```python
from build123d import *

# Parameters (mm, degrees)
SKETCH_1_R      = 2.15
EXTRUDE_1_DEPTH = 6


with BuildPart() as part:
    # 草图1 → 凸台-拉伸1 (new body)
    with BuildSketch(Plane.XY):
        with BuildLine():
            ThreePointArc((-43.896896246, -8.75), (-40.93656063, -9.720556733), (-39.12549448, -12.255434783))
            ThreePointArc((-39.12549448, -12.255434783), (41, 0), (-39.12549448, 12.255434783))
            ThreePointArc((-39.12549448, 12.255434783), (-40.93656063, 9.720556733), (-43.896896246, 8.75))
            Line((-43.896896246, 8.75), (-52, 8.75))
            Line((-52, 8.75), (-52, 30))
            Line((-52, 30), (-47.54, 30))
            ThreePointArc((-47.54, 30), (-44.004466094, 31.464466094), (-42.54, 35))
            Line((-42.54, 35), (-42.54, 37.5))
            ThreePointArc((-42.54, 37.5), (-38.982425028, 42.287422066), (-33.372235985, 40.262198963))
            ThreePointArc((-33.372235985, 40.262198963), (-30.171244586, 38.118753147), (-26.396349665, 38.887436588))
            ThreePointArc((-26.396349665, 38.887436588), (0, 47), (26.396349665, 38.887436588))
            ThreePointArc((26.396349665, 38.887436588), (30.171244586, 38.118753147), (33.372235985, 40.262198963))
            ThreePointArc((33.372235985, 40.262198963), (38.674773042, 42.369526686), (42.499484755, 38.135225128))
            Line((42.499484755, 38.135225128), (46.619156699, 5.971116201))
            ThreePointArc((46.619156699, 5.971116201), (47, 0), (46.619156699, -5.971116201))
            Line((46.619156699, -5.971116201), (42.499484755, -38.135225128))
            ThreePointArc((42.499484755, -38.135225128), (38.674773042, -42.369526686), (33.372235985, -40.262198963))
            ThreePointArc((33.372235985, -40.262198963), (30.171244586, -38.118753147), (26.396349665, -38.887436588))
            ThreePointArc((26.396349665, -38.887436588), (0, -47), (-26.396349665, -38.887436588))
            ThreePointArc((-26.396349665, -38.887436588), (-30.171244586, -38.118753147), (-33.372235985, -40.262198963))
            ThreePointArc((-33.372235985, -40.262198963), (-38.982425028, -42.287422066), (-42.54, -37.5))
            Line((-42.54, -37.5), (-42.54, -35))
            ThreePointArc((-42.54, -35), (-44.004466094, -31.464466094), (-47.54, -30))
            Line((-47.54, -30), (-52, -30))
            Line((-52, -30), (-52, -8.75))
            Line((-52, -8.75), (-43.896896246, -8.75))
        make_face()
        with Locations((37.54, -37.5)):
            Circle(SKETCH_1_R, mode=Mode.SUBTRACT)
        with Locations((-37.54, -37.5)):
            Circle(SKETCH_1_R, mode=Mode.SUBTRACT)
        with Locations((-37.54, 37.5)):
            Circle(SKETCH_1_R, mode=Mode.SUBTRACT)
        with Locations((37.54, 37.5)):
            Circle(SKETCH_1_R, mode=Mode.SUBTRACT)
    extrude(amount=EXTRUDE_1_DEPTH)


solid = part.part
```
The model under review builds one solid part; all positions refer to its coordinate system, in mm. A direction names the side the tool comes from. Give positions to 0.01 mm unless a question says otherwise; leave off trailing zeros. Write each loop counter-clockwise with the first axis right and the second up, starting at its lowest first coordinate (ties: lowest second). Pieces come first, ordered by that corner, then holes. Notation, with made-up numbers: (-36.5, -2.5) -> (16.5, -2.5) arc R28 ccw to (16.5, 20.5) -> close; hole circle Ø9 at (65.25, -0.75). An arc over 180 degrees is marked (long way). Answer in a Markdown table with one row per item.
1) Tool access review of faces 1 (the flat face through (-48, -8.75, 3)), 2 (the flat face through (-50, -30, 3)), 3 (the cylindrical face through (-40.972, -9.694, 2.958)): name each direction out of +Z, -Z, +X, -X, +Y, -Y from which nothing blocks a thin tool from reaching the whole face with its end or side.
Worked answers:
| item | result |
|---|---|
| face 1 | +Z, -Z, -X |
| face 2 | +Z, -Z, -X, -Y |
| face 3 | +Z, -Z |
2) Add section A-A on z = 4. Count the separate pieces of the cut face and the enclosed holes in it, plus the area to 3 significant figures.
Worked answers:
| item | result |
|---|---|
| separate pieces | 1 |
| enclosed holes | 4 |
| area | 2,510 mm² |
3) Add section B-B on x = 0. State the section outline as (y, z) points, plus the area to 3 significant figures.
Worked answers:
| item | result |
|---|---|
| outline | (-47, 0) -> (-41, 0) -> (-41, 6) -> (-47, 6) -> close; (41, 0) -> (47, 0) -> (47, 6) -> (41, 6) -> close |
| area | 72.0 mm² |
4) Add section D-D on x = 37.54. State the section outline as (y, z) points.
Worked answers:
| item | result |
|---|---|
| outline | (-42.5, 0) -> (-39.65, 0) -> (-39.65, 6) -> (-42.5, 6) -> close; (-35.35, 0) -> (-16.48, 0) -> (-16.48, 6) -> (-35.35, 6) -> close; (16.48, 0) -> (35.35, 0) -> (35.35, 6) -> (16.48, 6) -> close; (39.65, 0) -> (42.5, 0) -> (42.5, 6) -> (39.65, 6) -> close |
5) Clearance check with flat-ended pins moving along their axes: P1, Ø1, axis at x = 17, z = 1, coming from the +Y side; P2, Ø1.3, axis at x = -49, z = 2, coming from the +Y side; P3, Ø3, axis at x = -46.5, z = 3.5, coming from the +Y side. State where each tip first meets the part, or that it passes through.
Worked answers:
| item | result |
|---|---|
| P1 | y = 44.01 |
| P2 | y = 30 |
| P3 | y = 30.69 |
6) For L1, parallel to Y at x = 0, z = 1.9; L2, parallel to Y at x = 37.54, z = 4.65; L3, parallel to Y at x = -39.5, z = 1.5, list the stretches that pass through material, from the lowest coordinate up. Write a range as [from, to].
Worked answers:
| item | result |
|---|---|
| L1 | [-47, -41], [41, 47] |
| L2 | [-42.5, -39.65], [-35.35, -16.48], [16.48, 35.35], [39.65, 42.5] |
| L3 | [-42.1, -38.38], [-36.62, -11.37], [11.37, 36.62], [38.38, 42.1] |
7) Add section C-C on y = -11. State the section outline as (x, z) points.
Worked answers:
| item | result |
|---|---|
| outline | (-52, 0) -> (-39.72, 0) -> (-39.72, 6) -> (-52, 6) -> close; (39.5, 0) -> (45.98, 0) -> (45.98, 6) -> (39.5, 6) -> close |
8) Mouldability with a two-part tool opening along Y and no side actions: class faces 4 (the flat face through (-39, 14, 6)), 5 (the cylindrical face through (40.968, -1.629, 2.958)), 6 (the flat face through (44.588, -21.828, 2.958)), 7 (the cylindrical face through (37.26, 39.63, 2.96)) as +Y half, -Y half, draft (parallel to the pull), parting line (faces both ways), or undercut.
Worked answers:
| item | result |
|---|---|
| face 4 | draft |
| face 5 | undercut |
| face 6 | -Y half |
| face 7 | undercut |
